```python
from build123d import *

# Parameters (mm, degrees)
SKETCH1_W                       = 21
SKETCH1_H                       = 7
BOSS_EXTRUDE1_DEPTH             = 2
SKETCH4_W                       = 3.5
SKETCH4_H                       = 3
BOSS_EXTRUDE2_DEPTH             = 3
BOSS_EXTRUDE3_REACH             = 14.145
BOSS_EXTRUDE3_DIRECTION_2_REACH = 14.145


with BuildPart() as part:
    # Sketch1 → Boss-Extrude1 (new body)
    with BuildSketch(Plane(origin=(0, 0, 0), x_dir=(1, 0, 0), z_dir=(0, 1, 0))):
        Rectangle(SKETCH1_W, SKETCH1_H)
    extrude(amount=BOSS_EXTRUDE1_DEPTH)

    # Cut-Loft1: read off the stored shape, not the designer's step
    # Cut-Loft1: loft between two sections, ruled curve by curve
    cut_loft1_from = [
        Edge.make_bspline([(-8.811086142, 2, 2.515942564), (-13.842971271, 2, -1.106229719), (-10.220798987, 2, -6.138114848), (-5.188913858, 2, -2.515942564), (-0.157028729, 2, 1.106229719), (-3.779201013, 2, 6.138114848), (-8.811086142, 2, 2.515942564)], [0, 0, 0, 0, 0.5, 0.5, 0.5, 1, 1, 1, 1], 3, [1, 0.333333333, 0.333333333, 1, 0.333333333, 0.333333333, 1]),
    ]
    cut_loft1_to = [
        Edge.make_bspline([(-7.221614309, 0, 1.3823484), (-9.986311108, 0, 0.939119783), (-9.543082491, 0, -1.825577017), (-6.778385691, 0, -1.3823484), (-4.013688892, 0, -0.939119783), (-4.456917509, 0, 1.825577017), (-7.221614309, 0, 1.3823484)], [0, 0, 0, 0, 0.5, 0.5, 0.5, 1, 1, 1, 1], 3, [1, 0.333333333, 0.333333333, 1, 0.333333333, 0.333333333, 1]),
    ]
    cut_loft1 = Solid(Shell([*[Face.make_surface_from_curves(cut_loft1_from[k], cut_loft1_to[k]) for k in range(1)], Face(Wire(cut_loft1_from)), Face(Wire(cut_loft1_to))]))
    add(cut_loft1, mode=Mode.SUBTRACT)

    # Mirror1: Cut-Loft1 across plane
    add(cut_loft1.mirror(Plane(origin=(0, 0, 0), x_dir=(0, 0, 1), z_dir=(1, 0, 0))), mode=Mode.SUBTRACT)

    # Sketch4 → Boss-Extrude2 (add)
    with BuildSketch(Plane(origin=(0, 2, 0), x_dir=(1, 0, 0), z_dir=(0, 1, 0))):
        Rectangle(SKETCH4_W, SKETCH4_H)
    extrude(amount=BOSS_EXTRUDE2_DEPTH)

    # Boss-Extrude3: up to this face of the body (flat: up to its plane)
    boss_extrude3_end = Plane(part.part.faces().sort_by_distance((0, 3.5, 1.5))[0])
    # Sketch5 → Boss-Extrude3 (add, up to the picked face)
    with BuildSketch(Plane.XY, mode=Mode.PRIVATE) as boss_extrude3_sk1:
        Polygon((-2.6, 5), (-2.6, 6), (-1.3, 7.3), (1.3, 7.3), (2.6, 6), (2.6, 5), align=None)
    boss_extrude3_tool1 = split(extrude(boss_extrude3_sk1.sketch, amount=BOSS_EXTRUDE3_REACH, mode=Mode.PRIVATE), bisect_by=boss_extrude3_end, keep=Keep.BOTH, mode=Mode.PRIVATE)
    add(boss_extrude3_tool1.solids().sort_by(Axis((0, 6.032068, 0), (0, 0, 1)))[0])

    # Boss-Extrude3 direction 2: up to this face of the body (flat: up to its plane)
    boss_extrude3_direction_2_end = Plane(part.part.faces().sort_by_distance((0, 3.5, -1.5))[0])
    # Sketch5 → Boss-Extrude3 direction 2 (add, up to the picked face)
    with BuildSketch(Plane.XY, mode=Mode.PRIVATE) as boss_extrude3_direction_2_sk1:
        Polygon((-2.6, 5), (-2.6, 6), (-1.3, 7.3), (1.3, 7.3), (2.6, 6), (2.6, 5), align=None)
    boss_extrude3_direction_2_tool1 = split(extrude(boss_extrude3_direction_2_sk1.sketch, amount=-BOSS_EXTRUDE3_DIRECTION_2_REACH, mode=Mode.PRIVATE), bisect_by=boss_extrude3_direction_2_end, keep=Keep.BOTH, mode=Mode.PRIVATE)
    add(boss_extrude3_direction_2_tool1.solids().sort_by(Axis((0, 6.032068, 0), (0, 0, -1)))[0])


solid = part.part
```
The listing builds one solid part. Answer for the finished solid, in the listing's coordinates (mm). A direction names the side the tool comes from. Coordinates: 2 decimals unless noted, no trailing zeros. Write each loop counter-clockwise with the first axis right and the second up, starting at its lowest first coordinate (ties: lowest second). Pieces come first, ordered by that corner, then holes. Notation, with made-up numbers: (-12.75, 77) -> (31.25, 77) arc R29 ccw to (31.25, 106) -> close; hole circle Ø1 at (66.25, 32). An arc over 180 degrees is marked (long way). Write each question's results on one line, items separated by ' | '. Start each with the question number.
1) A cutting plane is placed at C-C (z = -1). Count the separate pieces of the cut face and the enclosed holes in it, then the cut area to 3 significant figures.
2) A tool of negligible diameter and unlimited length cuts with its end or side. For faces 4 (the flat face through (0, 5, 1.5)), 5 (the flat face through (2.6, 5.5, 0)), 6 (the flat face through (1.75, 3, 0)), 7 (the flat face through (0, 5, -1.5)), from which of +Z, -Z, +X, -X, +Y, -Y can it reach the whole face along a straight path? Write none if from no direction.
3) Straight lines are drawn through the part: probe 1 along Z at (x, y) = (-1, 5); probe 2 along Y at (x, z) = (-0.75, 2.75); probe 3 along X at (y, z) = (5.5, -0.75). For each, find the intervals that lie inside material, in ascending order.
4) A cutting plane is placed at A-A (x = 0.75). Determine the outline of the cut face in (y, z).
5) Flat-ended cylindrical pins translate along their axes: pin 1 Ø0.8 at (y, z) = (5.5, -0.5) entering from -X; pin 2 Ø1.5 at (y, z) = (3.5, -0.5) entering from +X; pin 3 Ø1.5 at (y, z) = (4, 0.5) entering from -X. Find the tip coordinate at first contact, or state that the pin passes through.
6) For a pull along Y with two mould halves and no side action, classify faces 1 (the flat face through (10.5, 1, 0)), 2 (the flat face through (1.9, 6.7, 0)), 3 (the flat face through (-2, 5, 0)) as +Y half, -Y half, draft (parallel to the pull), parting line (faces both ways), or undercut.
7) A cutting plane is placed at B-B (y = 5.75). Determine the outline of the cut face in (x, z).
Values follow:
1) separate pieces: 3 | enclosed holes: 0 | area: 47.1 mm²
2) face 4: +Z, +X, -X, +Y | face 5: +Z, -Z, +X, +Y | face 6: +Z, -Z, +X | face 7: -Z, +X, -X, +Y
3) probe 1: -1.5 to 1.5 | probe 2: 0 to 2 | probe 3: -2.6 to 2.6
4) outline: (0, -3.5) -> (2, -3.5) -> (2, -1.5) -> (7.3, -1.5) -> (7.3, 1.5) -> (2, 1.5) -> (2, 3.5) -> (0, 3.5) -> close
5) pin 1: x = -2.6 | pin 2: x = 1.75 | pin 3: x = -1.75
6) face 1: draft | face 2: +Y half | face 3: undercut
7) outline: (-2.6, -1.5) -> (2.6, -1.5) -> (2.6, 1.5) -> (-2.6, 1.5) -> close
